```python
from build123d import *

# Parameters (mm, degrees)
BOSS_EXTRUDE1_DEPTH = 70
CUT_EXTRUDE2_DEPTH  = 32


with BuildPart() as part:
    # Sketch1 → Boss-Extrude1 (new body)
    with BuildSketch(Plane(origin=(0, 0, 0), x_dir=(0, 0, -1), z_dir=(1, 0, 0))):
        with BuildLine():
            Line((-47, 0), (0, 0))
            Line((0, 0), (0, -47))
            ThreePointArc((0, -47), (-33.234018716, -33.234018716), (-47, 0))
        make_face()
    extrude(amount=BOSS_EXTRUDE1_DEPTH)

    # Sketch3 → Cut-Extrude2 (cut)
    with BuildSketch(Plane(origin=(0, 0, 47), x_dir=(-1, 0, 0), z_dir=(0, 0, -1))):
        Polygon((-15, 0), (-70, -20), (-70, 0), align=None)
    extrude(amount=CUT_EXTRUDE2_DEPTH, mode=Mode.SUBTRACT)


solid = part.part
```
Can you work these out from the model? Positions are in its coordinate system, mm. A direction names the side the tool comes from. Coordinates: 2 decimals unless noted, no trailing zeros. Loops run counter-clockwise (first coordinate to the right, second up) from the corner with the lowest first, then second, coordinate; pieces in that order, holes last. Notation, with made-up numbers: M 62,71.25 L 74,71.25 A18 ccw 74,93.25 Z; hole C -23.75,-35.75 d10. An arc over 180 degrees is marked long. Put each result on its own line as item: value. Start each with the question number.
(1) Imagine slicing it at C-C on x = 53.5. List the corners of the cut face in (y, z) for me, and give its area (3 significant figures).
(2) Imagine slicing it at D-D on y = -18. List the corners of the cut face in (x, z) for me.
(3) Will these pins go through, and if not, where does the flat tip stop? pin 1 Ø1 at (x, z) = (24.5, 22.5) entering from -Y; pin 2 Ø3 at (x, z) = (11.5, 33.5) entering from -Y; pin 3 Ø5 at (x, y) = (18.5, -16.5) entering from +Z.
(4) Imagine slicing it at A-A on z = 26. List the corners of the cut face in (x, y) for me.
(5) I need wall thicknesses on probe 1 along Z at (x, y) = (61, -12); probe 2 along Z at (x, y) = (25, -20); probe 3 along Y at (x, z) = (64, 16). Which ranges of each line are inside material? Lowest first, please.
(6) Imagine slicing it at B-B on y = -9.5. List the corners of the cut face in (x, z) for me (3 decimals), and give its area (3 significant figures).
(7) Which directions (+Z, -Z, +X, -X, +Y, -Y) give clear straight access to the entire face, cutting with the end or side of a thin tool? Please do faces 1 (the face through (42.12, -9.86, 31.22)), 2 (the face through (35, -23, 0)).
Worked answers:
1. outline: M -47,0 L 0,0 L 0,15 L -14,15 L -14,44.87 A47 ccw Z
1. area: 1,300 mm2
2. outline: M 0,0 L 70,0 L 70,15 L 64.5,15 L 64.5,43.42 L 0,43.42 Z
3. pin 1: stops at y = -41.53
3. pin 2: stops at y = -34.42
3. pin 3: stops at z = 44.87
4. outline: M 0,-39.15 L 70,-39.15 L 70,-20 L 15,0 L 0,0 Z
5. probe 1: z = 0 to 15
5. probe 2: z = 0 to 42.53
5. probe 3: y = -44.19 to -17.82
6. outline: M 0,0 L 70,0 L 70,15 L 41.125,15 L 41.125,46.03 L 0,46.03 Z
6. area: 2,330 mm2
7. face 1: +Z, +X, +Y
7. face 2: -Z, +X, -X, +Y, -Y
